Geometry check sheet. Reference: the model listing, model coordinates, mm. A direction names the side the tool comes from. Round coordinates to 2 decimals unless told otherwise and drop trailing zeros. Write each loop counter-clockwise with the first axis right and the second up, starting at its lowest first coordinate (ties: lowest second). Pieces come first, ordered by that corner, then holes. Notation, with made-up numbers: (4, -7) -> (30, -7) arc R17 ccw to (30, -3) -> close; hole circle Ø4 at (-39.75, 78.25). An arc over 180 degrees is marked (long way). Use a Markdown table: item, result.
```python
from build123d import *

# Parameters (mm, degrees)
PAD_DEPTH       = 19
POCKET_DEPTH    = 11.62232
POCKET002_DEPTH = 1.501
POCKET003_DEPTH = 1.501


with BuildPart() as part:
    # Sketch → Pad (new body)
    with BuildSketch(Plane.XY):
        with BuildLine():
            Line((0, 0), (16, 0))
            ThreePointArc((16, 0), (17.959845, 0.389838), (19.62132, 1.500001))
            Line((19.62132, 1.500001), (30.935023, 12.813715))
            ThreePointArc((30.935023, 12.813715), (32.045185, 14.475191), (32.435022, 16.435035))
            Line((32.435022, 32.435035), (32.435022, 16.435035))
            Line((30.935022, 32.435035), (32.435022, 32.435035))
            Line((30.935022, 16.435035), (30.935022, 32.435035))
            ThreePointArc((29.874363, 13.874375), (30.659366, 15.049216), (30.935022, 16.435035))
            Line((29.874363, 13.874375), (18.56066, 2.560661))
            ThreePointArc((16, 1.5), (17.385819, 1.775657), (18.56066, 2.560661))
            Line((16, 1.5), (0, 1.5))
            Line((0, 1.5), (0, 0))
        make_face()
    extrude(amount=PAD_DEPTH)

    # Sketch004 → Pocket (cut, through all)
    with BuildSketch(Plane(origin=(8.000009, -8.000001, 0), x_dir=(-0.707106, -0.707107, 0), z_dir=(-0.707107, 0.707106, 0))):
        Polygon((-28.935023, 17.3), (-25.435023, 17.3), (-25.435023, 16.5), (-20.435023, 16.5), (-20.435023, 17.3), (-16.935023, 17.3), (-16.935023, 16.5), (-15.935023, 16.5), (-15.935023, 15.5), (-15.135024, 15.5), (-15.135024, 12), (-15.935023, 12), (-15.935023, 7), (-15.135024, 7), (-15.135024, 3.5), (-15.935023, 3.5), (-15.935023, 2.5), (-16.935023, 2.5), (-16.935023, 1.7), (-20.435023, 1.7), (-20.435023, 2.5), (-25.435023, 2.5), (-25.435023, 1.7), (-28.935023, 1.7), (-28.935023, 2.5), (-29.935023, 2.5), (-29.935023, 3.5), (-30.735024, 3.5), (-30.735024, 7), (-29.935023, 7), (-29.935023, 12), (-30.735024, 12), (-30.735024, 15.5), (-29.935023, 15.5), (-29.935023, 16.5), (-28.935023, 16.5), align=None)
    extrude(amount=-POCKET_DEPTH, mode=Mode.SUBTRACT)

    # Sketch004001 → Pocket002 (cut, through all)
    with BuildSketch(Plane(origin=(30.935022, 0, 0), x_dir=(0, -1, 0), z_dir=(-1, 0, 0))):
        Polygon((-30.435035, 17.3), (-26.935035, 17.3), (-26.935035, 16.5), (-21.935035, 16.5), (-21.935035, 17.3), (-18.435035, 17.3), (-18.435035, 16.5), (-17.435035, 16.5), (-17.435035, 15.5), (-16.635036, 15.5), (-16.635036, 12), (-17.435035, 12), (-17.435035, 7), (-16.635036, 7), (-16.635036, 3.5), (-17.435035, 3.5), (-17.435035, 2.5), (-18.435035, 2.5), (-18.435035, 1.7), (-21.935035, 1.7), (-21.935035, 2.5), (-26.935035, 2.5), (-26.935035, 1.7), (-30.435035, 1.7), (-30.435035, 2.5), (-31.435035, 2.5), (-31.435035, 3.5), (-32.235036, 3.5), (-32.235036, 7), (-31.435035, 7), (-31.435035, 12), (-32.235036, 12), (-32.235036, 15.5), (-31.435035, 15.5), (-31.435035, 16.5), (-30.435035, 16.5), align=None)
    extrude(amount=-POCKET002_DEPTH, mode=Mode.SUBTRACT)

    # Sketch004001001 → Pocket003 (cut, through all)
    with BuildSketch(Plane(origin=(0, 1.5, 0), x_dir=(-1, 0, 0), z_dir=(0, 1, 0))):
        Polygon((-14, 17.3), (-10.5, 17.3), (-10.5, 16.5), (-5.5, 16.5), (-5.5, 17.3), (-2, 17.3), (-2, 16.5), (-1, 16.5), (-1, 15.5), (-0.200001, 15.5), (-0.200001, 12), (-1, 12), (-1, 7), (-0.200001, 7), (-0.200001, 3.5), (-1, 3.5), (-1, 2.5), (-2, 2.5), (-2, 1.7), (-5.5, 1.7), (-5.5, 2.5), (-10.5, 2.5), (-10.5, 1.7), (-14, 1.7), (-14, 2.5), (-15, 2.5), (-15, 3.5), (-15.800001, 3.5), (-15.800001, 7), (-15, 7), (-15, 12), (-15.800001, 12), (-15.800001, 15.5), (-15, 15.5), (-15, 16.5), (-14, 16.5), align=None)
    extrude(amount=-POCKET003_DEPTH, mode=Mode.SUBTRACT)


with BuildPart() as part_1:
    # Clone placement: moved
    add(part.part.moved(Location((2.38, -2.38, 19))))


solid = part_1.part
```
(1) Section check A-A on y = 27.5. Record the cut outline in (x, z), plus the area to 3 significant figures.
A:
| item | result |
|---|---|
| outline | (33.32, 19) -> (34.82, 19) -> (34.82, 20.7) -> (33.32, 20.7) -> close; (33.32, 36.3) -> (34.82, 36.3) -> (34.82, 38) -> (33.32, 38) -> close |
| area | 5.10 mm2 |
(2) Section check C-C on x = 7. Record the cut outline in (y, z), plus the area to 3 significant figures.
A:
| item | result |
|---|---|
| outline | (-2.38, 19) -> (-0.88, 19) -> (-0.88, 20.7) -> (-2.38, 20.7) -> close; (-2.38, 36.3) -> (-0.88, 36.3) -> (-0.88, 38) -> (-2.38, 38) -> close |
| area | 5.10 mm2 |
(3) Release check for a two-part mould opening along X. For faces 1 (the face through (22.171, 0.365, 28.535)), 2 (the face through (34.1, 15.6, 35.5)), 3 (the face through (2.58, -2, 33)), 4 (the face through (17, -2, 21.5)) record: +X half, -X half, draft (parallel to the pull), parting line (faces both ways), or undercut.
A:
| item | result |
|---|---|
| face 1 | +X half |
| face 2 | draft |
| face 3 | undercut |
| face 4 | undercut |
(4) Gauge pin test, flat ends, axial feed: pin 1 Ø1.5 at (x, z) = (26.5, 35) entering from +Y; pin 2 Ø3 at (x, z) = (6.5, 22) entering from +Y; pin 3 Ø2 at (x, z) = (31.5, 22) entering from +Y. Record the tip position at first contact, or that the pin passes through.
A:
| item | result |
|---|---|
| pin 1 | stops at y = 6.3 |
| pin 2 | stops at y = -0.88 |
| pin 3 | stops at y = 11.77 |
(5) Section check D-D on z = 30.5. Record the cut outline in (x, y), plus the area to 3 significant figures.
A:
| item | result |
|---|---|
| outline | (2.38, -2.38) -> (3.38, -2.38) -> (3.38, -0.88) -> (2.38, -0.88) -> close; (17.38, -2.38) -> (18.38, -2.38) arc R5.12 ccw to (22, -0.88) -> (22.71, -0.17) -> (21.65, 0.89) -> (20.94, 0.18) arc R3.62 cw to (18.38, -0.88) -> (17.38, -0.88) -> close; (31.55, 10.79) -> (32.61, 9.73) -> (33.32, 10.43) arc R5.12 ccw to (34.82, 14.06) -> (34.82, 15.06) -> (33.32, 15.06) -> (33.32, 14.06) arc R3.62 cw to (32.25, 11.49) -> close; (33.32, 29.06) -> (34.82, 29.06) -> (34.82, 30.06) -> (33.32, 30.06) -> close |
| area | 19.3 mm2 |
(6) Section check B-B on z = 24.5. Record the cut outline in (x, y), plus the area to 3 significant figures.
A:
| item | result |
|---|---|
| outline | (2.38, -2.38) -> (2.58, -2.38) -> (2.58, -0.88) -> (2.38, -0.88) -> close; (18.18, -2.38) -> (18.38, -2.38) arc R5.12 ccw to (22, -0.88) -> (22.14, -0.74) -> (21.08, 0.32) -> (20.94, 0.18) arc R3.62 cw to (18.38, -0.88) -> (18.18, -0.88) -> close; (32.11, 11.35) -> (33.17, 10.29) -> (33.32, 10.43) arc R5.12 ccw to (34.82, 14.06) -> (34.82, 14.26) -> (33.32, 14.26) -> (33.32, 14.06) arc R3.62 cw to (32.25, 11.49) -> close; (33.32, 29.86) -> (34.82, 29.86) -> (34.82, 30.06) -> (33.32, 30.06) -> close |
| area | 12.1 mm2 |
(7) Access from +Z, -Z, +X, -X, +Y, -Y to the whole of each face (thin tool, end or side, straight path). Record for faces 5 (the face through (18, -2, 26)), 6 (the face through (34, 15.055, 22)), 7 (the face through (32, 11, 31)), 8 (the face through (22, 0, 22.5)).
A:
| item | result |
|---|---|
| face 5 | +Y, -Y |
| face 6 | +X, -X |
| face 7 | -X, -Y |
| face 8 | +X, +Y |
(8) Thickness scan on line 1 (Y direction, x = 8.5, z = 36.75); line 2 (X direction, y = 14, z = 31); line 3 (Y direction, x = 33.5, z = 23.75). Record the ranges inside material, lowest first.
A:
| item | result |
|---|---|
| line 1 | y = -2.38 to -0.88 |
| line 2 | x = 33.31 to 34.81 |
| line 3 | y = 10.63 to 14.26, 29.86 to 30.06 |
